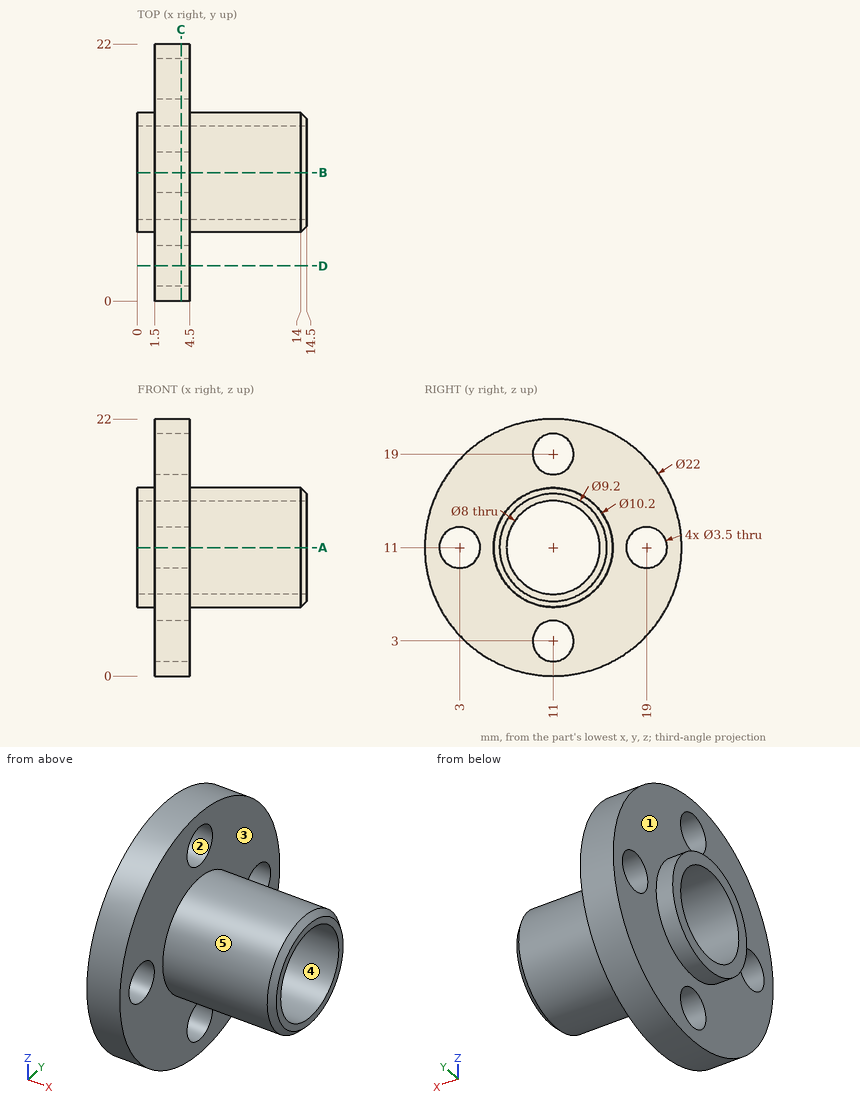
Could you check a few things on this drawing? It's one solid part, dimensions in mm from its lowest x, y, z. A direction names the side the tool comes from. Give positions to 0.01 mm unless a question says otherwise; leave off trailing zeros. Write each loop counter-clockwise with the first axis right and the second up, starting at its lowest first coordinate (ties: lowest second). Pieces come first, ordered by that corner, then holes.
(1) If I drill on L1, parallel to Y at x = 2.45, z = 11; L2, parallel to Z at x = 2.5, y = 11.25; L3, parallel to X at y = 13.75, z = 16.25, over which ranges is the centre line in solid material (lowest first)?
Output values:
L1: y = 0 to 1.25, 4.75 to 7, 15 to 17.25, 20.75 to 22
L2: z = 0 to 1.27, 4.73 to 7.01, 14.99 to 17.27, 20.73 to 22
L3: x = 1.5 to 4.5
(2) Thinking about a two-plate mould opening in Z: for the marked faces 3, 4 and 5, which applies, pulls with the +Z half, pulls with the -Z half, needs draft (parallel to the pull), parting line crosses it, or undercut?
Output values:
face 3: needs draft
face 4: undercut
face 5: parting line crosses it
(3) Imagine slicing it at C-C, the plane x = 3.75. Write out the boundary of the cut face in (y, z).
Output values:
outline: circle Ø22 at (11, 11); hole circle Ø3.5 at (3, 11); hole circle Ø8 at (11, 11); hole circle Ø3.5 at (11, 3); hole circle Ø3.5 at (11, 19); hole circle Ø3.5 at (19, 11)
(4) Imagine slicing it at A-A, the plane z = 11. Write out the boundary of the cut face in (x, y), and give its area (4 significant figures).
Output values:
outline: (0, 5.9) - (1.5, 5.9) - (1.5, 4.75) - (4.5, 4.75) - (4.5, 5.9) - (14, 5.9) - (14.5, 6.4) - (14.5, 7) - (0, 7) - close; (0, 15) - (14.5, 15) - (14.5, 15.6) - (14, 16.1) - (4.5, 16.1) - (4.5, 17.25) - (1.5, 17.25) - (1.5, 16.1) - (0, 16.1) - close; (1.5, 0) - (4.5, 0) - (4.5, 1.25) - (1.5, 1.25) - close; (1.5, 20.75) - (4.5, 20.75) - (4.5, 22) - (1.5, 22) - close
area: 46.05 mm2
(5) Will these pins go through, and if not, where does the flat tip stop? pin 1 (6 mm diameter, centred on x = 7, z = 7.5, fed in from +Y); pin 2 (4.5 mm diameter, centred on y = 11, z = 19, fed in from +X); pin 3 (3 mm diameter, centred on x = 4, y = 19.5, fed in from +Z); pin 4 (3 mm diameter, centred on y = 3, z = 11, fed in from +X).
Output values:
pin 1: stops at y = 21.84
pin 2: stops at x = 4.5
pin 3: stops at z = 19.49
pin 4: passes through
(6) On a 3-axis mill with a long thin cutter (end or side, diameter ignored), from which of +Z, -Z, +X, -X, +Y, -Y can I reach the whole of each face in a straight line? I mean the marked faces 1 and 2. Say none if no direction works.
Output values:
face 1: -X
face 2: +X, -X
(7) Imagine slicing it at D-D, the plane y = 3. Write out the boundary of the cut face in (x, z), and give its area (3 significant figures).
Output values:
outline: (1.5, 3.45) - (4.5, 3.45) - (4.5, 9.25) - (1.5, 9.25) - close; (1.5, 12.75) - (4.5, 12.75) - (4.5, 18.55) - (1.5, 18.55) - close
area: 34.8 mm2
